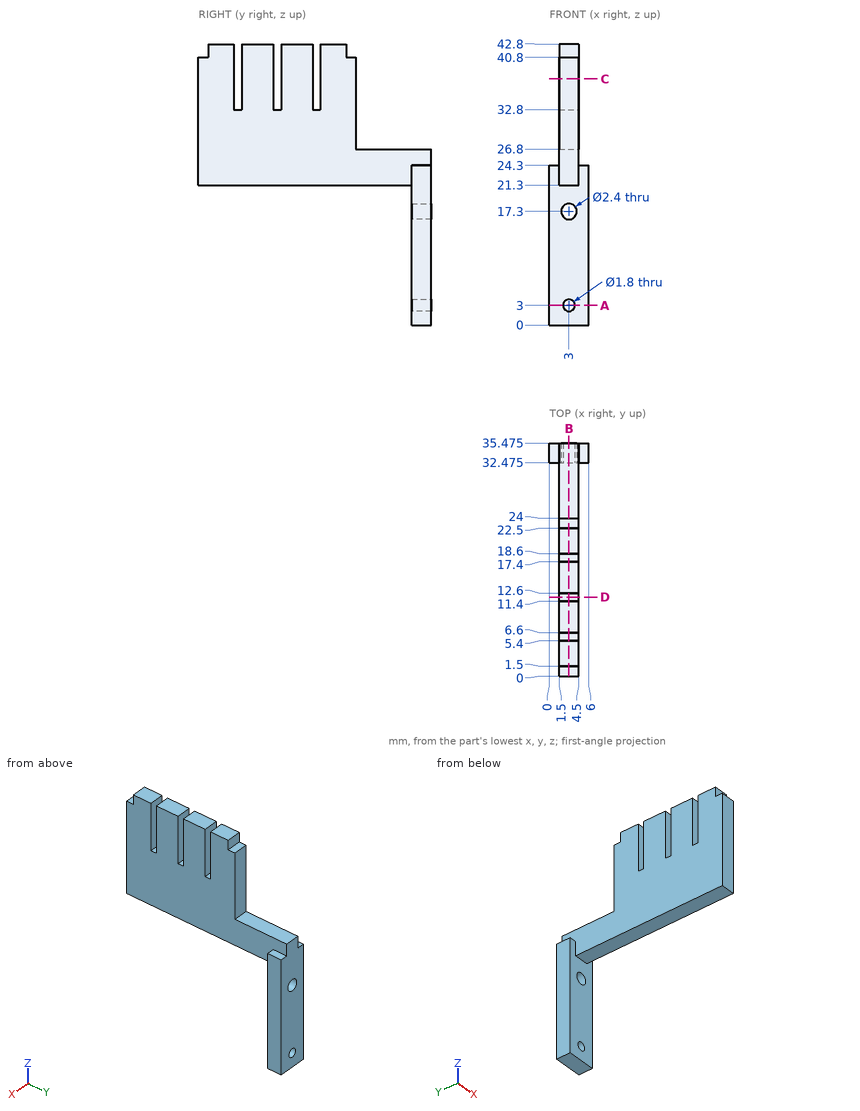
Geometry: see drawing. Coordinates: mm, zero at the bounding-box minimum. Give positions to 0.01 mm unless a question says otherwise; leave off trailing zeros. Write each loop counter-clockwise with the first axis right and the second up, starting at its lowest first coordinate (ties: lowest second). Pieces come first, ordered by that corner, then holes. Notation, with made-up numbers: M -27.5,46 L 15.5,46 A25 ccw 15.5,82 Z; hole C 23.5,-5.75 d11. An arc over 180 degrees is marked long. Answer in a Markdown table with one row per item. Add a question column.
(1) Section B-B on x = 3. State how many separate pieces and enclosed holes the cut face has, and give its area (3 significant figures).
(2) Section C-C on z = 37.5. Return loops of the section in (x, y).
(3) Section A-A on z = 3. Return loops of the section in (x, y) (3 decimals), and give its area (3 significant figures).
(4) First-contact query: pin 1 (3 mm diameter, centred on x = 3.5, y = 24.5, fed in from -Z); pin 2 (6.5 mm diameter, centred on y = 20.5, z = 36, fed in from -X); pin 3 (1.2 mm diameter, centred on x = 1, y = 34, fed in from +Z). Flat tips, straight axial feed; report the tip coordinate or a pass-through.
(5) Section D-D on y = 12. Return loops of the section in (x, z).
(6) Ray query, line 1 (Z direction, x = 3, y = 33.6); line 2 (Y direction, x = 4.15, z = 41.5); line 3 (X direction, y = 34, z = 3). Return the intervals inside material, ascending.
Result set:
| question | item | result |
|---|---|---|
| 1 | separate pieces | 3 |
| 1 | enclosed holes | 0 |
| 1 | area | 588 mm^2 |
| 2 | outline | M 1.5,0 L 4.5,0 L 4.5,5.4 L 1.5,5.4 Z; M 1.5,6.6 L 4.5,6.6 L 4.5,11.4 L 1.5,11.4 Z; M 1.5,12.6 L 4.5,12.6 L 4.5,17.4 L 1.5,17.4 Z; M 1.5,18.6 L 4.5,18.6 L 4.5,24 L 1.5,24 Z |
| 3 | outline | M 0,32.475 L 2.1,32.475 L 2.1,35.475 L 0,35.475 Z; M 3.9,32.475 L 6,32.475 L 6,35.475 L 3.9,35.475 Z |
| 3 | area | 12.6 mm^2 |
| 4 | pin 1 | stops at z = 21.3 |
| 4 | pin 2 | stops at x = 1.5 |
| 4 | pin 3 | stops at z = 26.8 |
| 5 | outline | M 1.5,21.3 L 4.5,21.3 L 4.5,32.8 L 1.5,32.8 Z |
| 6 | line 1 | z = 0 to 2.1, 3.9 to 16.1, 18.5 to 26.8 |
| 6 | line 2 | y = 1.5 to 5.4, 6.6 to 11.4, 12.6 to 17.4, 18.6 to 22.5 |
| 6 | line 3 | x = 0 to 2.1, 3.9 to 6 |
